Build history of the part. All positions in model axes, mm. Face numbers are marked on the shaded views. A direction names the side the tool comes from. Round coordinates to 2 decimals unless told otherwise and drop trailing zeros. Write each loop counter-clockwise with the first axis right and the second up, starting at its lowest first coordinate (ties: lowest second). Pieces come first, ordered by that corner, then holes.
Item 1: Band-saw the part on A-A, the plane z = 19. Write the cut outline in (x, y), then the cut area to 3 significant figures.
Item 2: Mould opens along Y. For the marked faces 1, 2, 3 and 4 say: +Y half, -Y half, draft (parallel to the pull), parting line (faces both ways), or undercut.
Item 3: 3-axis set-ups, long thin cutter, end or side, ignore diameter. For the marked faces 5 and 6: which of +Z, -Z, +X, -X, +Y, -Y reach the whole face in a straight line?
Item 4: Band-saw the part on C-C, the plane y = -38.5. Write the cut outline in (x, z), then the cut area to 3 significant figures.
Item 5: Wall check: probe 1 along Y at (x, z) = (-25, 9); probe 2 along X at (y, z) = (-30, 9); probe 3 along Z at (x, y) = (-51.5, 12.5). Give the ranges that are in metal, low to high.
Item 6: Band-saw the part on B-B, the plane x = -24. Write the cut outline in (y, z), then the cut area to 3 significant figures.
Autodesk Fusion 360 part; units mm, degrees
sketch "Sketch1" plane through (0, 0, 0) normal (0, 0, 1) x (1, 0, 0) in component "Component"
  line L0 (70, 55) -> (-70, 55)
  line L1 (-70, 55) -> (-70, -55)
  line L2 (-70, -55) -> (70, -55)
  line L3 (70, -55) -> (70, 55)
  line L4 (70, 55) -> (-70, -55) construction
  line L5 (-70, 55) -> (70, -55) construction
  dimension "d1" = 140
  dimension "d2" = 110
extrude "Extrude1" add sketch "Sketch1" along normal blind 35 in component "Component"
sketch "Sketch3" plane through (0, 0, 35) normal (0, 0, 1) x (-1, 0, 0) in component "Component"
  line L0 (-70, 55) -> (-70, -55)
  line L1 (-70, -55) -> (70, -55)
  line L2 (70, -55) -> (70, 55)
  line L3 (70, 55) -> (-70, 55)
  line L4 (65, -50) -> (-65, -50)
  line L5 (-65, -50) -> (-65, 50)
  line L6 (-65, 50) -> (65, 50)
  line L7 (65, 50) -> (65, -50)
  line L8 (65, -50) -> (-65, 50) construction
  line L9 (-65, -50) -> (65, 50) construction
  dimension "d5" = 130
  dimension "d6" = 100
extrude "Extrude2" cut sketch "Sketch3" against normal up to surface (30 mm away) contours L4 L5 L6 L7 in component "Component"
fillet "Fillet1" radius 5 4 edges at (65, -50, 20) (65, 50, 20) (-65, 50, 20) (-65, -50, 20) in component "Component"
fillet "Fillet2" radius 5 4 edges at (-70, 55, 17.5) (-70, -55, 17.5) (70, -55, 17.5) (70, 55, 17.5) in component "Component"
component "Component" placed x (1, 0, 0) y (0, 1, 0) z (0, 0, 1) at (0, 0, 0)
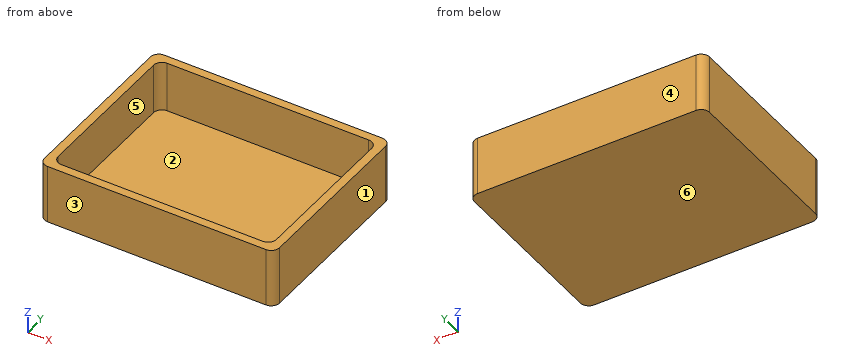
Results:
1. outline: (-70, -50) arc R5 ccw to (-65, -55) - (65, -55) arc R5 ccw to (70, -50) - (70, 50) arc R5 ccw to (65, 55) - (-65, 55) arc R5 ccw to (-70, 50) - close; hole (-65, -45) arc R5 ccw to (-60, -50) - (60, -50) arc R5 ccw to (65, -45) - (65, 45) arc R5 ccw to (60, 50) - (-60, 50) arc R5 ccw to (-65, 45) - close
1. area: 2,400 mm2
2. face 1: draft
2. face 2: undercut
2. face 3: -Y half
2. face 4: +Y half
3. face 5: +Z
3. face 6: -Z, +X, -X, +Y, -Y
4. outline: (-70, 0) - (70, 0) - (70, 35) - (65, 35) - (65, 5) - (-65, 5) - (-65, 35) - (-70, 35) - close
4. area: 1,000 mm2
5. probe 1: y = -55 to -50, 50 to 55
5. probe 2: x = -70 to -65, 65 to 70
5. probe 3: z = 0 to 5
6. outline: (-55, 0) - (55, 0) - (55, 35) - (50, 35) - (50, 5) - (-50, 5) - (-50, 35) - (-55, 35) - close
6. area: 850 mm2
